from build123d import *

# Parameters (mm, degrees)
CIRCLE001_R        = 41.5
EXTRUSION002_DEPTH = 10
EXTRUSION_DEPTH    = 10
CIRCLE_R           = 41.5
EXTRUSION001_DEPTH = 10
EXTRUSION003_DEPTH = 10


with BuildPart() as extrusion002:
    # Circle001 (on Cut009001_solid) → Extrusion002 (new body)
    with BuildSketch(Plane(origin=(-7.416555, 0.315657, 15), x_dir=(1, 0, 0), z_dir=(0, 0, 1))):
        Circle(CIRCLE001_R)
    extrude(amount=-EXTRUSION002_DEPTH)


with BuildPart() as extrusion:
    # Wire → Extrusion (new body)
    with BuildSketch(Plane(origin=(-7.75138, 65.661741, 15), x_dir=(1, 0, 0), z_dir=(0, 0, -1))):
        Polygon((0, 0), (-8.816291, 8.816291), (-5.098214, 22.403339), (5.346978, 19.539573), align=None)
    extrude(amount=EXTRUSION_DEPTH)


with BuildPart() as fusion:
    # Circle (on Cut009001_solid) → Extrusion001 (new body)
    with BuildSketch(Plane(origin=(53.009071, 0.089991, 15), x_dir=(1, 0, 0), z_dir=(0, 0, 1))):
        Circle(CIRCLE_R)
    extrude(amount=-EXTRUSION001_DEPTH)

    # Fusion: union Extrusion002, Extrusion
    add(extrusion002.part)
    add(extrusion.part)


with BuildPart() as fusion001:
    # Ellipse002 → Extrusion003 (new body)
    with BuildSketch(Plane(origin=(22.469609, 10.829601, 15), x_dir=(1, 0, 0), z_dir=(0, 0, 1))):
        with BuildLine():
            add(Edge.make_bspline(
                [(69, 0), (69, 65.817931), (-34.5, 32.908965), (-138, 0), (-34.5, -32.908965), (69, -65.817931), (69, 0)],
                knots=[0, 0, 0, 2.094395, 2.094395, 4.18879, 4.18879, 6.283185, 6.283185, 6.283185], degree=2, weights=[1, 0.5, 1, 0.5, 1, 0.5, 1]))
        make_face()
    extrude(amount=-EXTRUSION003_DEPTH)

    # Fusion001: union Fusion
    add(fusion.part)


solid = fusion001.part
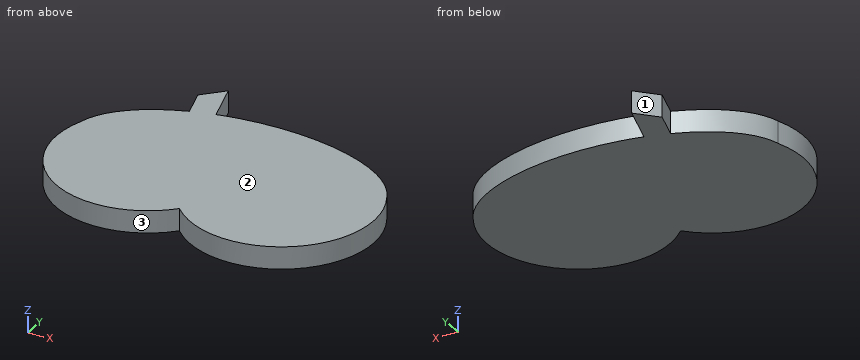
Work out the finished part from the listing and answer in its coordinate system (mm). Face numbers are marked on the shaded views. Round coordinates to 2 decimals unless told otherwise and drop trailing zeros. Loops run counter-clockwise (first coordinate to the right, second up) from the corner with the lowest first, then second, coordinate; pieces in that order, holes last. Notation, with made-up numbers: (25, 26.25) - (80, 26.25) arc R23 cw to (80, 54.25) - close; hole circle Ø7 at (38, -9). An arc over 180 degrees is marked (long way). Use one line per item in the form item = value. Start each with the question number.
(1) Consider line 1 (X direction, y = 0, z = 9); line 2 (X direction, y = -34, z = 9.75); line 3 (Y direction, x = 60.5, z = 11.5). Determine where each line is inside the solid, lowest interval first.
(2) Find section A-A on y = 10.5. Determine the outline of the cut face in (x, z).
(3) Determine the mould class of the marked faces 1, 2 and 3 for opening direction X: +X half, -X half, draft (parallel to the pull), parting line (faces both ways), or undercut.
(4) Find section B-B on y = 54.5. Determine the outline of the cut face in (x, z).
(5) Flat-ended cylindrical pins translate along their axes: P1, Ø4, axis at y = 35, z = 8, coming from the -X side; P2, Ø1, axis at y = 30, z = 11, coming from the +X side; P3, Ø4, axis at y = -22.5, z = 13.5, coming from the -X side. Find the tip coordinate at first contact, or state that the pin passes through.
Answer list:
q1.line_1 = -48.92 to 94.51
q1.line_2 = -30.76 to 15.92, 29.34 to 76.68
q1.line_3 = -40.73 to 42.54
q2.outline = (-47.65, 5) - (93.18, 5) - (93.18, 15) - (-47.65, 15) - close
q3.face_1 = -X half
q3.face_2 = draft
q3.face_3 = undercut
q4.outline = (-15.93, 5) - (-4.7, 5) - (-4.7, 15) - (-15.93, 15) - close
q5.P1 = -33.57
q5.P2 = 82.57
q5.P3 = -43.32
